```python
from build123d import *

# Parameters (mm, degrees)
SKETCH2_R          = 19
BASECIRCLE_DEPTH   = 5
CUT_EXTRUDE2_DEPTH = 8
CUT_EXTRUDE1_DEPTH = 10
CIRPATTERN1_COUNT  = 12


with BuildPart() as part:
    # Sketch2 → BaseCircle (new, symmetric)
    with BuildSketch(Plane.XY.offset(8)):
        with Locations((25, 25)):
            Circle(SKETCH2_R)
    extrude(amount=BASECIRCLE_DEPTH, both=True)

    # Sketch4 → Cut-Extrude2 (cut)
    with BuildSketch(Plane.XY.offset(13)):
        with BuildLine():
            Line((27.753960784, 26.59), (27.753960784, 23.41))
            ThreePointArc((27.753960784, 23.41), (21.82, 25), (27.753960784, 26.59))
        make_face()
    extrude(amount=-CUT_EXTRUDE2_DEPTH, mode=Mode.SUBTRACT)

    # Sketch3 → Cut-Extrude1 (cut)
    with BuildSketch(Plane.XY.offset(13)):
        with BuildLine():
            Line((20.082438143, 6.647409301), (23.705904774, 15.170370869))
            ThreePointArc((23.705904774, 15.170370869), (25, 15), (26.294095226, 15.170370869))
            Line((26.294095226, 15.170370869), (29.917561857, 6.647409301))
            ThreePointArc((29.917561857, 6.647409301), (25, 6), (20.082438143, 6.647409301))
        make_face()
    cut_extrude1 = extrude(amount=-CUT_EXTRUDE1_DEPTH, mode=Mode.SUBTRACT)

    # CirPattern1: Cut-Extrude1 ×12 about axis
    cirpattern1_axis = Axis((25, 25, 0), (0, 0, 1))
    for i in range(1, CIRPATTERN1_COUNT):
        add(cut_extrude1.rotate(cirpattern1_axis, i * 360 / CIRPATTERN1_COUNT), mode=Mode.SUBTRACT)


solid = part.part
```
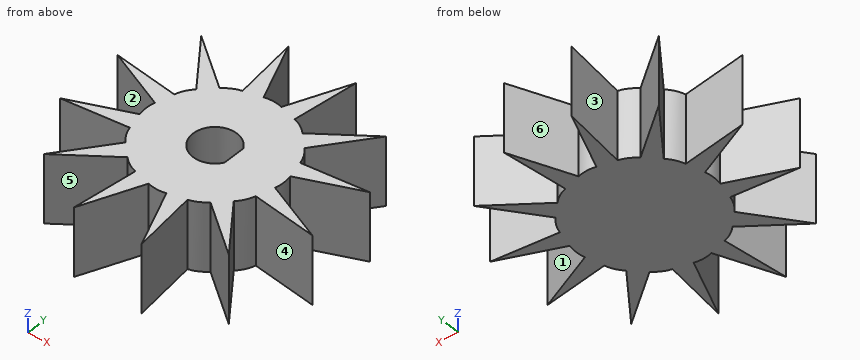
Could you check a few things on this model? Use its own coordinates, in mm. Face numbers are marked on the shaded views. A direction names the side the tool comes from. Coordinates: 2 decimals unless noted, no trailing zeros. Write each loop counter-clockwise with the first axis right and the second up, starting at its lowest first coordinate (ties: lowest second). Pieces come first, ordered by that corner, then holes. Notation, with made-up numbers: M -38,80 L -15,80 A13 ccw -15,90 Z; hole C 47.25,36.25 d3. An arc over 180 degrees is marked long. Answer as CSV lines item,"result". Start each with the question number.
1) Please list where these lines run through material, in increasing order: line 1 (Y direction, x = 25, z = 9.75); line 2 (X direction, y = 12, z = 3.5); line 3 (X direction, y = 24, z = 10.5). Write a range as from..to.
2) We'd pull the mould along Y, two halves only. Please class the marked faces 4, 5 and 6: +Y half, -Y half, draft (parallel to the pull), parting line (faces both ways), or undercut.
3) I want a section at D-D, the plane y = 25. Please give me the cut outline in (x, z), and give its area (3 significant figures).
4) For P1, Ø1, axis at x = 12, z = 5.5, coming from the +Y side (3 decimals); P2, Ø2.5, axis at y = 25.5, z = 10, coming from the -X side; P3, Ø1.5, axis at y = 27, z = 9, coming from the -X side, each with a flat end and sliding along its axis, tell me the tip position at first contact or that it passes through.
5) I want a section at C-C, the plane x = 25. Please give me the cut outline in (y, z), and give its area (3 significant figures).
6) I want a section at B-B, the plane y = 39. Please give me the cut outline in (x, z).
7) I want a section at A-A, the plane x = 16.5. Please give me the cut outline in (y, z), and give its area (3 significant figures).
8) For the marked faces 1, 2 and 3, which set-ups out of +Z, -Z, +X, -X, +Y, -Y let a thin tool reach every point of the face, with its end or its side?
Data:
1,line 1,"y = 15..21.82, 28.18..35"
1,line 2,"x = 11.89..12.14, 20.74..22.36, 27.64..29.26, 37.86..38.11"
1,line 3,"x = 15.1..21.98, 27.75..34.9"
2,face 4,"undercut"
2,face 5,"-Y half"
2,face 6,"+Y half"
3,outline,"M 15,3 L 35,3 L 35,13 L 27.75,13 L 27.75,5 L 21.82,5 L 21.82,13 L 15,13 Z"
3,area,"153 mm^2"
4,P1,"stops at y = 38.435"
4,P2,"stops at x = 14.1"
4,P3,"stops at x = 11.75"
5,outline,"M 15,3 L 35,3 L 35,13 L 28.18,13 L 28.18,5 L 21.82,5 L 21.82,13 L 15,13 Z"
5,area,"149 mm^2"
6,outline,"M 20.61,3 L 21.93,3 L 21.93,13 L 20.61,13 Z; M 28.07,3 L 29.39,3 L 29.39,13 L 28.07,13 Z"
7,outline,"M 15.28,3 L 18.12,3 L 18.12,13 L 15.28,13 Z; M 19.74,3 L 30.26,3 L 30.26,13 L 19.74,13 Z; M 31.88,3 L 34.72,3 L 34.72,13 L 31.88,13 Z"
7,area,"162 mm^2"
8,face 1,"+Z, -Z, +X"
8,face 2,"+Z, -Z, -X"
8,face 3,"+Z, -Z"
